from build123d import *

# Parameters (mm, degrees)
SKETCH1_R           = 5
BOSS_EXTRUDE1_DEPTH = 22.5
BOSS_EXTRUDE4_DEPTH = 10
BOSS_EXTRUDE5_DEPTH = 20
FILLET1_SIZE        = 20
BOSS_EXTRUDE6_DEPTH = 25
BOSS_EXTRUDE7_START = 30
BOSS_EXTRUDE7_DEPTH = 30
FILLET3_SIZE        = 20
SKETCH8_W           = 200
SKETCH8_H           = 240
BOSS_EXTRUDE8_DEPTH = 10
CHAMFER1_SIZE       = 10


# Some blends are built 0.0001 mm under size
with BuildPart() as part:
    # Sketch1 → Boss-Extrude1 (new, symmetric)
    with BuildSketch(Plane.XY):
        with Locations(Location((0, 180, 0), (0, 0, 180))):
            Circle(SKETCH1_R)
    extrude(amount=BOSS_EXTRUDE1_DEPTH, both=True)

    # Sketch4 → Boss-Extrude4 (add)
    with BuildSketch(Plane.XY.offset(22.5)):
        with BuildLine():
            Line((-20, 180), (-20, 205))
            Line((-20, 205), (20, 205))
            Line((20, 205), (20, 180))
            ThreePointArc((20, 180), (0, 160), (-20, 180))
        make_face()
    extrude(amount=BOSS_EXTRUDE4_DEPTH)

    # Sketch5 → Boss-Extrude5 (add)
    with BuildSketch(Plane.XY.offset(32.5)):
        with BuildLine():
            Line((-20, 180), (20, 180))
            ThreePointArc((20, 180), (0, 160), (-20, 180))
        make_face()
    extrude(amount=BOSS_EXTRUDE5_DEPTH)

    # Fillet1
    # a fillet whose section is not a circle: 20 mm, written as the material it takes off along each edge
    with BuildSketch(Plane(origin=(0, 180, 52.5), x_dir=(0.003141587485879206, 0.9999950652018581, 0), z_dir=(-0.9999950652018581, 0.003141587485879206, 0))) as fillet1_piece_1:
        with BuildLine():
            Bezier((20, FILLET1_SIZE), (20, 0), (20 - FILLET1_SIZE, 0), weights=[1, 0.707106781, 1])
            Line((20 - FILLET1_SIZE, 0), (20, 0))
            Line((20, 0), (20, FILLET1_SIZE))
        make_face()
    revolve(axis=Axis((0, 180, 52.5), (0, 0, -1)), revolution_arc=359.64, mode=Mode.SUBTRACT)

    # Sketch6 → Boss-Extrude6 (add)
    with BuildSketch(Plane(origin=(0, 180, 0), x_dir=(1, 0, 0), z_dir=(0, 1, 0))):
        with BuildLine():
            Line((20, -32.5), (-20, -32.5))
            ThreePointArc((-20, -32.5), (0, -52.5), (20, -32.5))
        make_face()
    extrude(amount=BOSS_EXTRUDE6_DEPTH)

    # Sketch7 → Boss-Extrude7 (add)
    with BuildSketch(Plane(origin=(0, 0, -22.5), x_dir=(-1, 0, 0), z_dir=(0, 0, -1)).offset(BOSS_EXTRUDE7_START)):
        with BuildLine():
            Line((20, 180), (20, 205))
            Line((20, 205), (-20, 205))
            Line((-20, 205), (-20, 180))
            ThreePointArc((-20, 180), (0, 160), (20, 180))
        make_face()
    extrude(amount=-BOSS_EXTRUDE7_DEPTH)

    # Fillet3
    # a fillet whose section is not a circle: 20 mm, written as the material it takes off along each edge
    with BuildSketch(Plane(origin=(0, 180, -52.5), x_dir=(1, 0, 0), z_dir=(0, 1, 0))) as fillet3_piece_1:
        with BuildLine():
            Bezier((20, -FILLET3_SIZE), (20, 0), (20 - FILLET3_SIZE, 0), weights=[1, 0.707106781, 1])
            Line((20 - FILLET3_SIZE, 0), (20, 0))
            Line((20, 0), (20, -FILLET3_SIZE))
        make_face()
    revolve(axis=Axis((0, 180, -52.5), (0, 0, -1)), revolution_arc=180, mode=Mode.SUBTRACT)
    with BuildSketch(Plane(origin=(20, 255, -52.5), x_dir=(-1, 0, 0), z_dir=(0, -1, 0))) as fillet3_piece_2:
        with BuildLine():
            Bezier((FILLET3_SIZE, 0), (0, 0), (0, -FILLET3_SIZE), weights=[1, 0.707106781, 1])
            Line((0, -FILLET3_SIZE), (0, 0))
            Line((0, 0), (FILLET3_SIZE, 0))
        make_face()
    extrude(amount=75, mode=Mode.SUBTRACT)
    with BuildSketch(Plane(origin=(-20, 180, -52.5), x_dir=(0, 0, 1), z_dir=(0, 1, 0))) as fillet3_piece_3:
        with BuildLine():
            Bezier((FILLET3_SIZE, 0), (0, 0), (0, FILLET3_SIZE), weights=[1, 0.707106781, 1])
            Line((0, FILLET3_SIZE), (0, 0))
            Line((0, 0), (FILLET3_SIZE, 0))
        make_face()
    extrude(amount=75, mode=Mode.SUBTRACT)

    # Sketch8 → Boss-Extrude8 (add)
    with BuildSketch(Plane(origin=(0, 205, 0), x_dir=(1, 0, 0), z_dir=(0, 1, 0))):
        Rectangle(SKETCH8_W, SKETCH8_H)
    extrude(amount=BOSS_EXTRUDE8_DEPTH)

    # Chamfer1
    chamfer1_edges = [part.edges().sort_by_distance(p)[0] for p in [
        (100, 205, 0),
        (0, 205, -120),
        (-100, 205, 0),
        (0, 205, 120),
    ]]
    chamfer(chamfer1_edges, length=CHAMFER1_SIZE - 0.0001)  # a hair under: the kernel refuses the full size


solid = part.part
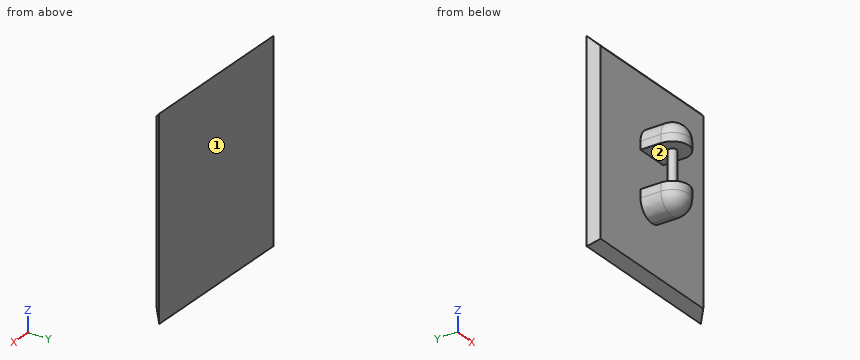
Build history of the part. All positions in model axes, mm. Face numbers are marked on the shaded views. Round coordinates to 2 decimals unless told otherwise and drop trailing zeros. Answer in a Markdown table with one row per item.
1. Mould opens along Z. For the marked faces 1 and 2 say: +Z half, -Z half, draft (parallel to the pull), parting line (faces both ways), or undercut.
Geometry check:
| item | result |
|---|---|
| face 1 | draft |
| face 2 | undercut |
2. Probe L1, parallel to Y at x = -78.5, z = -102.5; L2, parallel to X at y = 179.5, z = -27; L3, parallel to X at y = 207, z = 75. List the from-to ranges inside material, lowest first. Write a range as [from, to].
Geometry check:
| item | result |
|---|---|
| L1 | [205, 215] |
| L2 | [-19.99, 19.99] |
| L3 | [-92, 92] |
3. Flat gauge pins, fed straight in: P1, Ø3, axis at x = 32, y = 202, coming from the -Z side; P2, Ø5, axis at x = 13, y = 175.5, coming from the -Z side; P3, Ø3, axis at y = 195.5, z = 30, coming from the +X side; P4, Ø8, axis at y = 190, z = 25.5, coming from the -X side. Where does each tip first touch, or does it go through?
Geometry check:
| item | result |
|---|---|
| P1 | through |
| P2 | z = -49.03 |
| P3 | x = 20 |
| P4 | x = -20 |
